```python
from build123d import *

# Parameters (mm, degrees)
SKETCH1_W           = 28
SKETCH1_H           = 28
BOSS_EXTRUDE1_DEPTH = 10
SKETCH2_R           = 4.075
CUT_EXTRUDE1_DEPTH  = 23.181073013
CUT_EXTRUDE2_DEPTH  = 1


with BuildPart() as part:
    # Sketch1 → Boss-Extrude1 (new body)
    with BuildSketch(Plane(origin=(0, 0, 0), x_dir=(1, 0, 0), z_dir=(0, 1, 0))):
        Rectangle(SKETCH1_W, SKETCH1_H)
    extrude(amount=BOSS_EXTRUDE1_DEPTH)

    # Sketch2 → Cut-Extrude1 (cut, through all)
    with BuildSketch(Plane(origin=(0, 10, 0), x_dir=(1, 0, 0), z_dir=(0, 1, 0))):
        with Locations(Location((0, 0, 0), (0, 0, 270))):
            Circle(SKETCH2_R)
    extrude(amount=-CUT_EXTRUDE1_DEPTH, mode=Mode.SUBTRACT)

    # Sketch3 → Cut-Extrude2 (cut)
    with BuildSketch(Plane(origin=(0, 10, 0), x_dir=(1, 0, 0), z_dir=(0, 1, 0))):
        with BuildLine():
            Line((4.075, -2.440671014), (4.075, 2.440671014))
            ThreePointArc((4.075, 2.440671014), (-4.75, 0), (4.075, -2.440671014))
        make_face()
    extrude(amount=-CUT_EXTRUDE2_DEPTH, mode=Mode.SUBTRACT)


solid = part.part
```
The model under review builds one solid part; all positions refer to its coordinate system, in mm. A direction names the side the tool comes from. Coordinates: 2 decimals unless noted, no trailing zeros. Write each loop counter-clockwise with the first axis right and the second up, starting at its lowest first coordinate (ties: lowest second). Pieces come first, ordered by that corner, then holes.
1) Machinability: for faces 1 (the face through (4.075, 9.5, 0)), 2 (the face through (14, 5, 0)), which of the approach directions +Z, -Z, +X, -X, +Y, -Y give a long, thin tool a straight path to every point of the face, cutting with its end or side? Answer none if there is none.
2) The part is to be moulded in two halves that separate along X. For faces 3 (the face through (-14, 5, 0)), 4 (the face through (0, 5, -14)), 5 (the face through (-4, 9, 1.4)), 6 (the face through (-2.48, 4.563, -3.234)), say which applies: pulls with the +X half, pulls with the -X half, needs draft (parallel to the pull), parting line crosses it, or undercut.
3) We need section A-A on x = 0. State the section outline as (y, z) points (3 decimals), then the cut area to 3 significant figures.
4) We need section B-B on y = 7. State the section outline as (x, z) points (3 decimals).
5) We need section C-C on z = 1.25. State the section outline as (x, y) points (3 decimals), then the cut area to 3 significant figures.
6) To check wall thickness, follow probe 1 along X at (y, z) = (9.6, 0) (3 decimals); probe 2 along Z at (x, y) = (0, 9.55); probe 3 along X at (y, z) = (5.25, 0) (3 decimals). State the ranges of each line that lie inside material, in increasing order.
Answer list:
1. face 1: +Y
1. face 2: +Z, -Z, +X, +Y, -Y
2. face 3: pulls with the -X half
2. face 4: needs draft
2. face 5: undercut
2. face 6: undercut
3. outline: (0, -14) - (10, -14) - (10, -4.75) - (9, -4.75) - (9, -4.075) - (0, -4.075) - close; (0, 4.075) - (9, 4.075) - (9, 4.75) - (10, 4.75) - (10, 14) - (0, 14) - close
3. area: 197 mm2
4. outline: (-14, -14) - (14, -14) - (14, 14) - (-14, 14) - close; hole circle Ø8.15 at (0, 0)
5. outline: (-14, 0) - (-3.879, 0) - (-3.879, 9) - (-4.583, 9) - (-4.583, 10) - (-14, 10) - close; (3.879, 0) - (14, 0) - (14, 10) - (4.075, 10) - (4.075, 9) - (3.879, 9) - close
5. area: 202 mm2
6. probe 1: x = -14 to -4.75, 4.075 to 14
6. probe 2: z = -14 to -4.75, 4.75 to 14
6. probe 3: x = -14 to -4.075, 4.075 to 14
